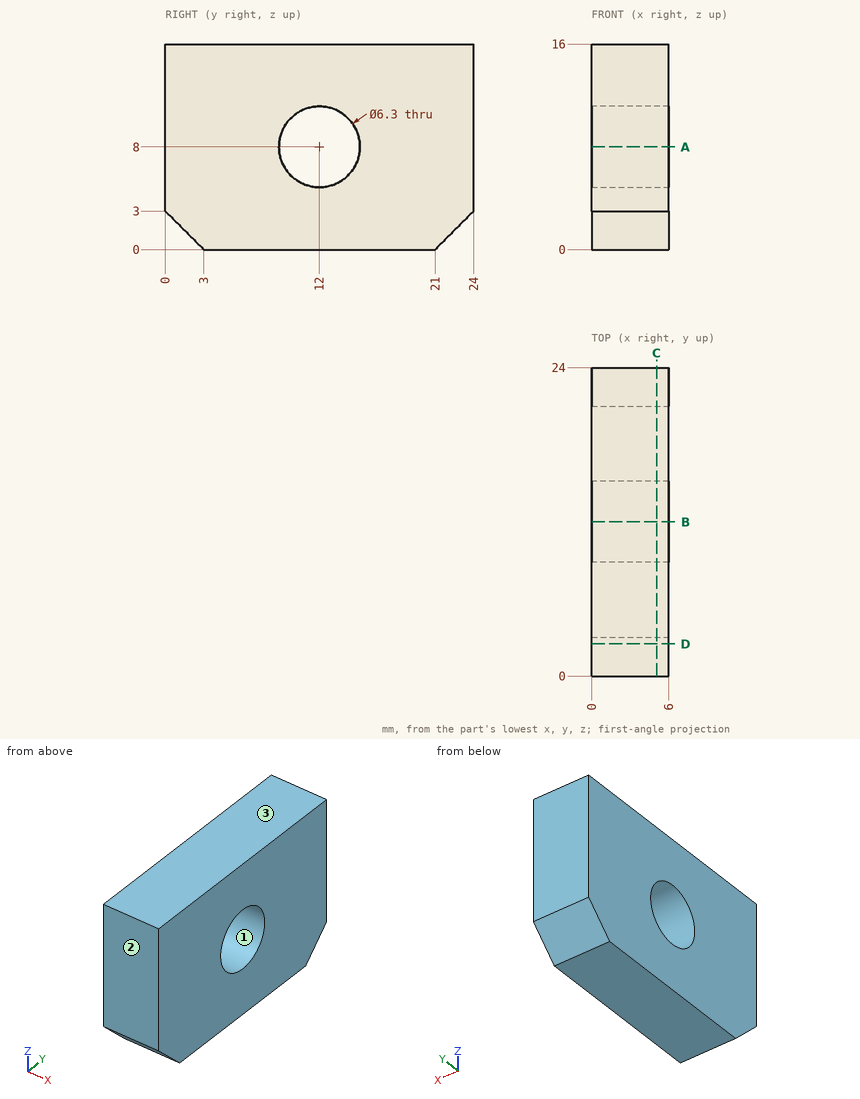
Verification items for this drawing (mm, ordinates from the low corner). Give positions to 0.01 mm unless a question says otherwise; leave off trailing zeros. Loops run counter-clockwise (first coordinate to the right, second up) from the corner with the lowest first, then second, coordinate; pieces in that order, holes last. Notation, with made-up numbers: M 86.25,72.25 L 113.25,72.25 A20 ccw 113.25,84.25 Z; hole C -23.75,-25.5 d10. An arc over 180 degrees is marked long. Write item = value, one per line. Start each with the question number.
1. Section check A-A, the plane z = 8. Enter the section's corners in (x, y).
2. Section check B-B, the plane y = 12. Enter the section's corners in (x, z).
3. Thickness scan on probe 1 along Y at (x, z) = (3.3, 8); probe 2 along Z at (x, y) = (2.95, 12); probe 3 along Y at (x, z) = (4.25, 9.75). Record the ranges inside material, lowest first.
4. Section check C-C, the plane x = 5.05. Enter the section's corners in (y, z), plus the area to 3 significant figures.
5. Section check D-D, the plane y = 2.5. Enter the section's corners in (x, z), plus the area to 3 significant figures.
6. Draft check along Z on the marked faces 1, 2 and 3. Enter one of: +Z half, -Z half, draft (parallel to the pull), parting line (faces both ways), or undercut.
Values follow:
q1.outline = M 0,0 L 6,0 L 6,8.85 L 0,8.85 Z; M 0,15.15 L 6,15.15 L 6,24 L 0,24 Z
q2.outline = M 0,0 L 6,0 L 6,4.85 L 0,4.85 Z; M 0,11.15 L 6,11.15 L 6,16 L 0,16 Z
q3.probe_1 = 0 to 8.85, 15.15 to 24
q3.probe_2 = 0 to 4.85, 11.15 to 16
q3.probe_3 = 0 to 9.38, 14.62 to 24
q4.outline = M 0,3 L 3,0 L 21,0 L 24,3 L 24,16 L 0,16 Z; hole C 12,8 d6.3
q4.area = 344 mm^2
q5.outline = M 0,0.5 L 6,0.5 L 6,16 L 0,16 Z
q5.area = 93.0 mm^2
q6.face_1 = undercut
q6.face_2 = draft
q6.face_3 = +Z half
